```python
from build123d import *

# Parameters (mm, degrees)
F2_DEPTH   = 3
F2_TAPER   = -3
F6_D       = 5
F6_ON_F4_D = 5


# Not quite as in the source:
# - the program builds the solid bodies; features that only make, move or delete a surface that nothing else refers to are left out


with BuildPart() as f2:
    # F0 (on Top) → F2 (new body)
    with BuildSketch(Plane.XY):
        Polygon((-13.9245763421, -24.6634986252), (9.9384738132, -24.6634986252), (9.9384738132, -13.1047982723), (29.8719406128, -13.1047982723), (29.8719406128, 46.2553314865), (13.0966929719, 64.9538859725), (-16.9530268759, 65.1064962149), (-35.7809066772, 47.6274192333), (-35.7809066772, -13.7434657663), (-13.9245763421, -13.7434657663), align=None)
    extrude(amount=F2_DEPTH, taper=F2_TAPER)

    # F6 (through all)
    with Locations(Plane(origin=(0, 0, 0), x_dir=(1, 0, 0), z_dir=(0, 0, -1))):
        with Locations((-15.4966376722, -52.7129508555), (7.3292911984, -52.3064211011), (7.3292911984, -38.3762717247), (7.3292911984, -17.4282062799), (-15.4966376722, 7.6540475711), (7.3292911984, 8.0594113097)):
            Hole(F6_D / 2)

    # F6 on F4 (through all)
    with Locations(Plane(origin=(0, 0, 0), x_dir=(1, 0, 0), z_dir=(0, 0, -1))):
        with Locations((-15.7919153571, -38.9971844852), (-15.7919153571, -18.486443907)):
            Hole(F6_ON_F4_D / 2)


solid = f2.part
```
Work out the finished part from the listing and answer in its coordinate system (mm). Give positions to 0.01 mm unless a question says otherwise; leave off trailing zeros. One line per item, written item: value. Start each with the question number.
1. Determine the mould class of faces 1 (the face through (-13.294, 38.887, 1.521)), 2 (the face through (-3, 20, 0)) for opening direction Y: released by +Y, released by -Y, zero draft, split by the parting line, or undercut.
2. Find section A-A (x = 6). State how many separate pieces and enclosed holes the cut face has, and give its area (3 significant figures).
3. This flat-tipped pin is pushed along its axis until it touches: P1, Ø1, axis at x = 17, z = 1.5, coming from the -Y side. Where does it stop, or does it pass through?
4. Find the intervals of material crossed by probe 1 along Y at (x, z) = (6.5, 1.15); probe 2 along X at (y, z) = (43, 2.7); probe 3 along X at (y, z) = (52, 1.65), in increasing order.
Reported:
1. face 1: undercut
1. face 2: zero draft
2. separate pieces: 5
2. enclosed holes: 0
2. area: 219 mm²
3. P1: stops at y = -13.21
4. probe 1: y = -24.72 to -10.42, -5.7 to 15.07, 19.79 to 36.02, 40.73 to 49.95, 54.66 to 65.05
4. probe 2: x = -35.92 to 30.01
4. probe 3: x = -31.2 to -17.89, -13.1 to 4.85, 9.81 to 24.83
